Work out the finished part from the listing and answer in its coordinate system (mm). A direction names the side the tool comes from. Round coordinates to 2 decimals unless told otherwise and drop trailing zeros. Loops run counter-clockwise (first coordinate to the right, second up) from the corner with the lowest first, then second, coordinate; pieces in that order, holes last. Notation, with made-up numbers: (21.5, 32.5) -> (55.5, 32.5) arc R15 ccw to (55.5, 44.5) -> close; hole circle Ø10 at (50, -28.75). An arc over 180 degrees is marked (long way). Use one line per item in the form item = value.
```python
from build123d import *

# Parameters (mm, degrees)
SKETCH2_W            = 102
SKETCH2_H            = 105
BOSS_EXTRUDE1_DEPTH  = 1.5
CUT_EXTRUDE1_DEPTH   = 10
CUT_EXTRUDE2_DEPTH   = 10
SKETCH5_W            = 3
SKETCH5_H            = 10
BOSS_EXTRUDE2_DEPTH  = 17
FILLET1_R            = 3
M3_CLEARANCE_HOLE1_D = 3.4
SKETCH8_W            = 3
SKETCH8_H            = 10
BOSS_EXTRUDE3_DEPTH  = 15
M3_CLEARANCE_HOLE2_D = 3.4
FILLET2_R            = 3
FILLET3_R            = 1
FILLET1_OF_MIRROR1_R = 3
M3_CLEARANCE_HOLE3_D = 3.2


with BuildPart() as part:
    # Sketch2 → Boss-Extrude1 (new, symmetric)
    with BuildSketch(Plane.XY):
        Rectangle(SKETCH2_W, SKETCH2_H)
    extrude(amount=BOSS_EXTRUDE1_DEPTH, both=True)

    # Sketch3 → Cut-Extrude1 (cut)
    with BuildSketch(Plane.XY.offset(1.5)):
        with BuildLine():
            Line((-20, 1), (20, 1))
            ThreePointArc((20, 1), (21, 0), (20, -1))
            Line((20, -1), (-20, -1))
            ThreePointArc((-20, -1), (-21, 0), (-20, 1))
        make_face()
        with BuildLine():
            Line((-20, 6), (20, 6))
            ThreePointArc((20, 6), (21, 5), (20, 4))
            Line((20, 4), (-20, 4))
            ThreePointArc((-20, 4), (-21, 5), (-20, 6))
        make_face()
        with BuildLine():
            Line((-20, 11), (20, 11))
            ThreePointArc((20, 11), (21, 10), (20, 9))
            Line((20, 9), (-20, 9))
            ThreePointArc((-20, 9), (-21, 10), (-20, 11))
        make_face()
        with BuildLine():
            Line((-20, 16), (20, 16))
            ThreePointArc((20, 16), (21, 15), (20, 14))
            Line((20, 14), (-20, 14))
            ThreePointArc((-20, 14), (-21, 15), (-20, 16))
        make_face()
        with BuildLine():
            Line((-20, 21), (20, 21))
            ThreePointArc((20, 21), (21, 20), (20, 19))
            Line((20, 19), (-20, 19))
            ThreePointArc((-20, 19), (-21, 20), (-20, 21))
        make_face()
    extrude(amount=-CUT_EXTRUDE1_DEPTH, mode=Mode.SUBTRACT)

    # Sketch4 → Cut-Extrude2 (cut)
    with BuildSketch(Plane.XY.offset(1.5)):
        Polygon((-19, -12.5), (24, -12.5), (24, -40.5), (-19, -40.5), (-24, -35), (-24, -18), align=None)
    extrude(amount=-CUT_EXTRUDE2_DEPTH, mode=Mode.SUBTRACT)

    # Sketch5 → Boss-Extrude2 (add)
    with BuildSketch(Plane(origin=(0, 0, -1.5), x_dir=(-1, 0, 0), z_dir=(0, 0, -1))):
        with Locations((49.5, -37.5)):
            Rectangle(SKETCH5_W, SKETCH5_H)
    boss_extrude2 = extrude(amount=BOSS_EXTRUDE2_DEPTH)

    # Fillet1
    fillet1_edges = [part.edges().sort_by_distance(p)[0] for p in [
        (-49.5, -32.5, -1.5),
        (-48, -37.5, -1.5),
        (-49.5, -42.5, -1.5),
    ]]
    fillet(fillet1_edges, radius=FILLET1_R)

    # M3 Clearance Hole1 (through all)
    with Locations(Plane.ZY.offset(51)):
        with Locations((-13.5, -37.5)):
            m3_clearance_hole1 = Hole(M3_CLEARANCE_HOLE1_D / 2)

    # Sketch8 → Boss-Extrude3 (add)
    with BuildSketch(Plane(origin=(0, 0, -1.5), x_dir=(-1, 0, 0), z_dir=(0, 0, -1))):
        with Locations((-42.58, -45.91)):
            Rectangle(SKETCH8_W, SKETCH8_H)
    extrude(amount=BOSS_EXTRUDE3_DEPTH)

    # M3 Clearance Hole2 (through all)
    with Locations(Plane(origin=(44.08, 0, 0), x_dir=(0, 0, -1), z_dir=(1, 0, 0))):
        with Locations((10.93, -45.91)):
            Hole(M3_CLEARANCE_HOLE2_D / 2)

    # Fillet2
    fillet2_edges = [part.edges().sort_by_distance(p)[0] for p in [
        (41.08, -45.91, -1.5),
        (42.58, -40.91, -1.5),
        (44.08, -45.91, -1.5),
    ]]
    fillet(fillet2_edges, radius=FILLET2_R)

    # Fillet3
    fillet3_edges = [part.edges().sort_by_distance(p)[0] for p in [
        (42.58, -50.91, -1.5),
    ]]
    fillet(fillet3_edges, radius=FILLET3_R)

    # Mirror1: Boss-Extrude2, M3 Clearance Hole1 across plane
    add(boss_extrude2.mirror(Plane.ZX))
    add(m3_clearance_hole1.mirror(Plane.ZX), mode=Mode.SUBTRACT)

    # Fillet1 of Mirror1
    fillet1_of_mirror1_edges = [part.edges().sort_by_distance(p)[0] for p in [
        (-49.5, 32.5, -1.5),
        (-48, 37.5, -1.5),
        (-49.5, 42.5, -1.5),
    ]]
    fillet(fillet1_of_mirror1_edges, radius=FILLET1_OF_MIRROR1_R)

    # M3 Clearance Hole3 (through all)
    with Locations(Plane(origin=(0, 0, -1.5), x_dir=(-1, 0, 0), z_dir=(0, 0, -1))):
        with Locations((-1, -6.5), (-1, -46.5)):
            Hole(M3_CLEARANCE_HOLE3_D / 2)


solid = part.part
```
(1) Find section C-C, the plane y = 41. Write down the section's boundary in (x, z), then the cut area to 3 significant figures.
Completed:
outline = (-51, -18.5) -> (-48, -18.5) -> (-48, -4.5) arc R3 cw to (-45, -1.5) -> (51, -1.5) -> (51, 1.5) -> (-51, 1.5) -> close
area = 359 mm2
(2) For a pull along Y with two mould halves and no side action, classify faces 1 (the cylindrical face through (42.52, -39.6, -2.02)), 2 (the flat face through (2, -12.5, 0)), 3 (the flat face through (-51, 0, -1)) as +Y half, -Y half, draft (parallel to the pull), parting line (faces both ways), or undercut.
Completed:
face_1 = +Y half
face_2 = undercut
face_3 = draft
(3) Find section D-D, the plane x = 1. State how many separate pieces and enclosed holes the cut face has, then the cut area to 3 significant figures.
Completed:
separate_pieces = 9
enclosed_holes = 0
area = 182 mm2
(4) Consider L1, parallel to Y at x = -49.75, z = -13.5; L2, parallel to Y at x = 42.9, z = -10.93; L3, parallel to X at y = -22, z = 0.75. Determine where each line is inside the solid, lowest interval first.
Completed:
L1 = -42.5 to -39.2, -35.8 to -32.5, 32.5 to 35.8, 39.2 to 42.5
L2 = -50.91 to -47.61, -44.21 to -40.91
L3 = -51 to -24, 24 to 51
(5) Given P1, Ø8, axis at y = -30, z = -8, coming from the -X side; P2, Ø2, axis at y = 33.5, z = -15.5, coming from the +X side; P3, Ø0.9, axis at x = 42.5, z = -7.5, coming from the +Y side; P4, Ø3.5, axis at x = 42, z = -6.5, coming from the -Y side, each flat-ended and moving along its own axis, determine where each tip first touches the part or whether it passes through.
Completed:
P1 = -51
P2 = -48
P3 = -40.91
P4 = -50.91
(6) Find section B-B, the plane y = -15.5. Write down the section's boundary in (x, z).
Completed:
outline = (-51, -1.5) -> (-21.73, -1.5) -> (-21.73, 1.5) -> (-51, 1.5) -> close; (24, -1.5) -> (51, -1.5) -> (51, 1.5) -> (24, 1.5) -> close
(7) Find section A-A, the plane x = 14. Write down the section's boundary in (y, z), then the cut area to 3 significant figures.
Completed:
outline = (-52.5, -1.5) -> (-40.5, -1.5) -> (-40.5, 1.5) -> (-52.5, 1.5) -> close; (-12.5, -1.5) -> (-1, -1.5) -> (-1, 1.5) -> (-12.5, 1.5) -> close; (1, -1.5) -> (4, -1.5) -> (4, 1.5) -> (1, 1.5) -> close; (6, -1.5) -> (9, -1.5) -> (9, 1.5) -> (6, 1.5) -> close; (11, -1.5) -> (14, -1.5) -> (14, 1.5) -> (11, 1.5) -> close; (16, -1.5) -> (19, -1.5) -> (19, 1.5) -> (16, 1.5) -> close; (21, -1.5) -> (52.5, -1.5) -> (52.5, 1.5) -> (21, 1.5) -> close
area = 201 mm2
(8) For faces 4 (the cylindrical face through (-48.71, -43.81, -2.02)), 5 (the flat face through (3, -40.5, 0)), 6 (the cylindrical face through (-48.71, 31.19, -2.02)), 7 (the flat face through (44.08, -46, -9)), determine the directions among +Z, -Z, +X, -X, +Y, -Y from which every point of the face is accessible in a straight line to the end or side of a thin tool.
Completed:
face_4 = -Z, -X, -Y
face_5 = +Z, -Z
face_6 = -Z, +X, -X
face_7 = -Z, +X, +Y, -Y
